Check sheet for the modelled part. Datum: model origin and axes. Units: mm. A direction names the side the tool comes from. Round coordinates to 2 decimals unless told otherwise and drop trailing zeros. Write each loop counter-clockwise with the first axis right and the second up, starting at its lowest first coordinate (ties: lowest second). Pieces come first, ordered by that corner, then holes. Notation, with made-up numbers: M 58.5,73.25 L 71.5,73.25 A35 ccw 71.5,108.25 Z; hole C 35.5,33 d9. An arc over 180 degrees is marked long. Answer in a Markdown table with one row per item.
```python
from build123d import *

# Parameters (mm, degrees)
BOSS_EXTRUDE1_DEPTH = 50


with BuildPart() as part:
    # Sketch4 → Boss-Extrude1 (new body, symmetric)
    with BuildSketch(Plane.XY):
        with BuildLine():
            Line((4.8, -20), (17.2, -20))
            ThreePointArc((17.2, -20), (19.179898987, -19.179898987), (20, -17.2))
            Line((20, -17.2), (20, -4.8))
            ThreePointArc((20, -4.8), (19.765685425, -4.234314575), (19.2, -4))
            Line((19.2, -4), (16.190663761, -4))
            ThreePointArc((16.190663761, -4), (15.624978336, -4.234314575), (15.390663761, -4.8))
            Line((15.390663761, -4.8), (15.390663761, -10.2))
            ThreePointArc((15.390663761, -10.2), (14.896810507, -10.939103626), (14.024978336, -10.765685425))
            Line((14.024978336, -10.765685425), (9.40588745, -6.146594539))
            ThreePointArc((9.40588745, -6.146594539), (8.365378244, -4.589362465), (8, -2.752481989))
            Line((8, -2.752481989), (8, 0))
            Line((8, 0), (3.5, 0))
            ThreePointArc((3.5, 0), (2.474873734, -2.474873734), (0, -3.5))
            Line((0, -3.5), (0, -8))
            Line((0, -8), (2.752481989, -8))
            ThreePointArc((2.752481989, -8), (4.589362465, -8.365378244), (6.146594539, -9.40588745))
            Line((6.146594539, -9.40588745), (10.765685425, -14.024978336))
            ThreePointArc((10.765685425, -14.024978336), (10.939103626, -14.896810507), (10.2, -15.390663761))
            Line((10.2, -15.390663761), (4.8, -15.390663761))
            ThreePointArc((4.8, -15.390663761), (4.234314575, -15.624978336), (4, -16.190663761))
            Line((4, -16.190663761), (4, -19.2))
            ThreePointArc((4, -19.2), (4.234314575, -19.765685425), (4.8, -20))
        make_face()
    extrude(amount=BOSS_EXTRUDE1_DEPTH, both=True)

    # Mirror1: part across plane


with BuildPart() as part_1:
    add(part.part)
    add(part.part.mirror(Plane(origin=(0, 0, 0), x_dir=(0, 0, 1), z_dir=(1, 0, 0))))

    # Mirror2: part across plane


with BuildPart() as part_2:
    add(part_1.part)
    add(part_1.part.mirror(Plane.ZX))


solid = part_2.part
```
1. Section check B-B, the plane y = 13. Record the cut outline in (x, z).
Found:
| item | result |
|---|---|
| outline | M -20,-50 L -9.74,-50 L -9.74,50 L -20,50 Z; M 9.74,-50 L 20,-50 L 20,50 L 9.74,50 Z |
2. Section check A-A, the plane y = -1. Record the cut outline in (x, z).
Found:
| item | result |
|---|---|
| outline | M -8,-50 L -3.35,-50 L -3.35,50 L -8,50 Z; M 3.35,-50 L 8,-50 L 8,50 L 3.35,50 Z |
3. Access from +Z, -Z, +X, -X, +Y, -Y to the whole of each face (thin tool, end or side, straight path). Record for faces 5 (the face through (18, 4, 1)), 6 (the face through (15.391, 7, 1)), 7 (the face through (-4, -18, 1)), 8 (the face through (11, 20, 1)), 9 (the face through (20, -11, 1)).
Found:
| item | result |
|---|---|
| face 5 | +Z, -Z, +X |
| face 6 | +Z, -Z |
| face 7 | +Z, -Z, -Y |
| face 8 | +Z, -Z, +X, -X, +Y |
| face 9 | +Z, -Z, +X, +Y, -Y |
4. Scan lines: L1, parallel to Y at x = -16, z = -42; L2, parallel to Y at x = -9.5, z = 2. Record each from-to range of solid material in increasing order.
Found:
| item | result |
|---|---|
| L1 | y = -20 to -4.02, 4.02 to 20 |
| L2 | y = -20 to -15.39, -12.76 to -6.24, 6.24 to 12.76, 15.39 to 20 |
5. Draft check along Y on faces 1 (the face through (-8.376, -4.614, 0.7)), 2 (the face through (-19.16, -19.2, 0.7)), 3 (the face through (-8, 0, 1)), 4 (the face through (-19.16, 19.2, 0.7)). Enter one of: +Y half, -Y half, draft (parallel to the pull), parting line (faces both ways), or undercut.
Found:
| item | result |
|---|---|
| face 1 | undercut |
| face 2 | -Y half |
| face 3 | undercut |
| face 4 | +Y half |
6. Go/stop test with flat-tipped pins: pin 1 (4.5 mm diameter, centred on y = -0.5, z = -24.5, fed in from +X); pin 2 (3 mm diameter, centred on x = 0, z = 21, fed in from +Y); pin 3 (0.9 mm diameter, centred on y = -18, z = -20.5, fed in from -X). Record where each tip stops, or that it passes through.
Found:
| item | result |
|---|---|
| pin 1 | stops at x = 8 |
| pin 2 | stops at y = 8 |
| pin 3 | stops at x = -19.98 |
